Can you work these out from the model? Positions are in its coordinate system, mm. Face numbers are marked on the shaded views. A direction names the side the tool comes from. Coordinates: 2 decimals unless noted, no trailing zeros. Order: outer loops, then holes, each group sorted by start corner. A loop starts at its lowest first (then second) coordinate and runs counter-clockwise, first axis right, second up. Notation, with made-up numbers: (24, -32.75) -> (75, -32.75) arc R20 ccw to (75, -26.75) -> close; hole circle Ø2 at (23, -28). An arc over 180 degrees is marked (long way). Answer in a Markdown table with one row per item. Add a question column.
1. Imagine slicing it at C-C on z = 0. Write out the boundary of the cut face in (x, y).
2. On a 3-axis mill with a long thin cutter (end or side, diameter ignored), from which of +Z, -Z, +X, -X, +Y, -Y can I reach the whole of each face in a straight line? I mean the marked faces 3 and 4. Say none if no direction works.
3. We'd pull the mould along X, two halves only. Please class the marked faces 1 and 2: pulls with the +X half, pulls with the -X half, needs draft (parallel to the pull), parting line crosses it, or undercut.
4. If I drill on line 1 along Y through (x, z) = (0, -3); line 2 along Y through (x, z) = (0, -0.95); line 3 along Y through (x, z) = (-20, 3), over which ranges is the centre line in solid material (lowest first)? Write a range as [from, to].
5. Will these pins go through, and if not, where does the flat tip stop? pin 1 (1.5 mm diameter, centred on y = 21, z = -1.5, fed in from -X); pin 2 (2 mm diameter, centred on x = 26, z = 0, fed in from -Y); pin 3 (1.5 mm diameter, centred on x = 23.5, y = -9.5, fed in from +Z); pin 4 (1.5 mm diameter, centred on x = 13, y = 25, fed in from +Z).
from build123d import *

# Parameters (mm, degrees)
SKETCH1_R           = 32.5
SKETCH1_R_2         = 25
BOSS_EXTRUDE1_DEPTH = 3.5
SKETCH2_R           = 31
SKETCH2_R_2         = 26.75
CUT_EXTRUDE1_DEPTH  = 1
CHAMFER1_SIZE       = 1


with BuildPart() as part:
    # Sketch1 → Boss-Extrude1 (new, symmetric)
    with BuildSketch(Plane.XY):
        Circle(SKETCH1_R)
        Circle(SKETCH1_R_2, mode=Mode.SUBTRACT)
    extrude(amount=BOSS_EXTRUDE1_DEPTH, both=True)

    # Sketch2 → Cut-Extrude1 (cut)
    with BuildSketch(Plane.XY.offset(3.5)):
        Circle(SKETCH2_R)
        Circle(SKETCH2_R_2, mode=Mode.SUBTRACT)
    cut_extrude1 = extrude(amount=-CUT_EXTRUDE1_DEPTH, mode=Mode.SUBTRACT)

    # Mirror1: Cut-Extrude1 across plane
    add(cut_extrude1.mirror(Plane.XY), mode=Mode.SUBTRACT)

    # Chamfer1
    chamfer1_edges = [part.edges().sort_by_distance(p)[0] for p in [
        (-32.5, 0, -3.5),
        (-32.5, 0, 3.5),
        (-25, 0, -3.5),
        (-25, 0, 3.5),
    ]]
    chamfer(chamfer1_edges, length=CHAMFER1_SIZE)


solid = part.part
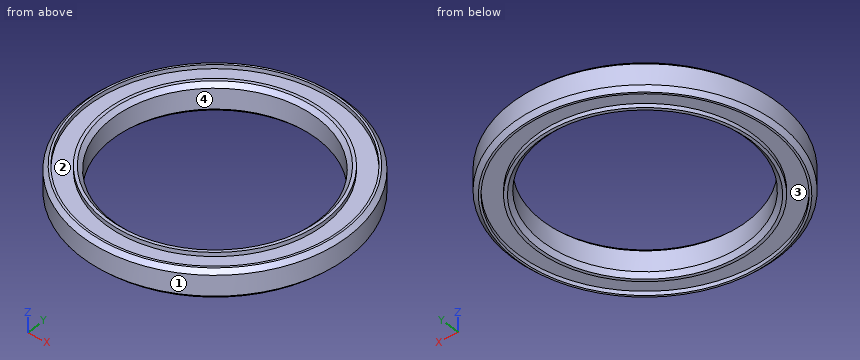
Answers follow:
| question | item | result |
|---|---|---|
| 1 | outline | circle Ø65 at (0, 0); hole circle Ø50 at (0, 0) |
| 2 | face 3 | -Z |
| 2 | face 4 | +Z, -Z |
| 3 | face 1 | parting line crosses it |
| 3 | face 2 | undercut |
| 4 | line 1 | y = [-32, -31], [-26.75, -25.5], [25.5, 26.75], [31, 32] |
| 4 | line 2 | y = [-32.5, -25], [25, 32.5] |
| 4 | line 3 | y = [-24.98, -23.69], [-17.76, -15.82], [15.82, 17.76], [23.69, 24.98] |
| 5 | pin 1 | stops at x = -25.42 |
| 5 | pin 2 | stops at y = -20.77 |
| 5 | pin 3 | stops at z = 3.5 |
| 5 | pin 4 | stops at z = 2.5 |
